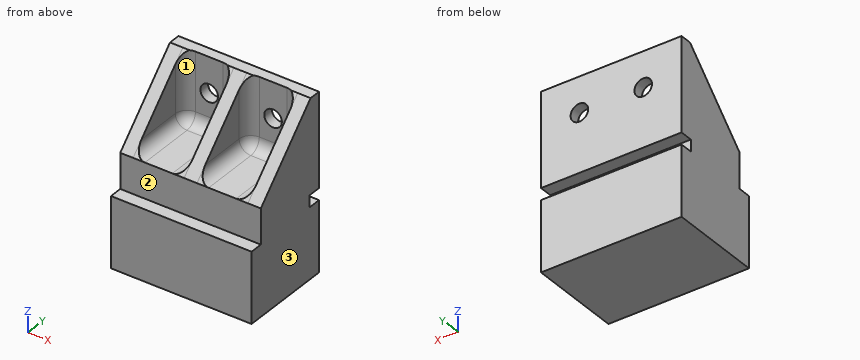
from build123d import *

# Parameters (mm, degrees)
F1_DEPTH     = 38.1
F2_W         = 13.81125
F2_H         = 19.05
F3_DEPTH     = 19.05
F4_T1_DEPTH  = 7.46125
F4_T3_DEPTH  = 7.46125
F4_S7_W      = 3.175
F4_S7_H      = 3.175
F4_T8_DEPTH  = 3.175
F4_S13_W     = 3.175
F4_S13_H     = 3.175
F4_T14_DEPTH = 3.175
F4_S19_W     = 3.175
F4_S19_H     = 3.175
F4_T20_DEPTH = 3.175
F4_S25_W     = 3.175
F4_S25_H     = 3.175
F4_T26_DEPTH = 3.175
F4_T32_DEPTH = 15.875
F4_T37_DEPTH = 15.875
F4_T42_DEPTH = 15.875
F4_T47_DEPTH = 15.875
F4_T52_DEPTH = 15.875
F4_T57_DEPTH = 15.875
F4_T62_DEPTH = 15.875
F4_T67_DEPTH = 15.875
F6_DEPTH     = 2.8585


# Not quite as in the source:
# - a fillet or chamfer that OpenCascade refuses, or shapes differently, is made with other operations: its cross-section is extruded or revolved along the edge and cut away or added


with BuildPart() as f1:
    # F0 (on Right) → F1 (new body)
    with BuildSketch(Plane.YZ):
        Polygon((0, 19.05), (0, 0), (25.4, 0), (25.4, 19.05), (21.9075, 19.05), (21.9075, 22.225), (25.4, 22.225), (25.4, 47.625), (22.225, 47.625), (22.225, 28.575), (3.4925, 28.575), (3.4925, 19.05), align=None)
        Polygon((22.225, 47.625), (3.4925, 28.575), (22.225, 28.575), align=None)
    extrude(amount=F1_DEPTH)

    # F2 (on face) → F3 (cut)
    with BuildSketch(Plane.XZ.offset(-3.4925)):
        with Locations((27.701875, 38.1)):
            Rectangle(F2_W, F2_H)
        with Locations((10.398125, 38.1)):
            Rectangle(F2_W, F2_H)
    extrude(amount=-F3_DEPTH, mode=Mode.SUBTRACT)

    # F4: fillet of radius 3.175 on 10 edges, made by hand

    # F4_s2 → F4_t1 (join)
    with BuildSketch(Plane.YZ.offset(6.6675)):
        with BuildLine():
            ThreePointArc((19.3675, 28.575), (21.6125640303, 29.5049359697), (22.5425, 31.75))
            Line((22.5425, 31.75), (22.5425, 28.575))
            Line((22.5425, 28.575), (19.3675, 28.575))
        make_face()
    extrude(amount=F4_T1_DEPTH)

    # F4_s4 → F4_t3 (join)
    with BuildSketch(Plane.YZ.offset(23.97125)):
        with BuildLine():
            ThreePointArc((19.3675, 28.575), (21.6125640303, 29.5049359697), (22.5425, 31.75))
            Line((22.5425, 31.75), (22.5425, 28.575))
            Line((22.5425, 28.575), (19.3675, 28.575))
        make_face()
    extrude(amount=F4_T3_DEPTH)


with BuildPart() as f4_tool6:
    # F4_s7 → F4_t8 (new body)
    with BuildSketch(Plane.YZ.offset(6.6675)):
        with Locations((20.955, 30.1625)):
            Rectangle(F4_S7_W, F4_S7_H)
    extrude(amount=-F4_T8_DEPTH)

    # F4_s9 → F4_t10 (revolve, cut)
    with BuildSketch(Plane(origin=(6.6675, 19.3675, 31.75), x_dir=(0, -0.7071067812, 0.7071067812), z_dir=(0, -0.7071067812, -0.7071067812))):
        with BuildLine():
            ThreePointArc((0, -3.175), (3.175, 0), (0, 3.175))
            Line((0, 3.175), (0, -3.175))
        make_face()
    revolve(axis=Axis((6.6675, 19.3675, 31.75), (-1, 0, 0)), mode=Mode.SUBTRACT)


with BuildPart() as f1_1:
    add(f1.part)

    # F4_t5: union F4_tool6
    add(f4_tool6.part)


with BuildPart() as f4_tool12:
    # F4_s13 → F4_t14 (new body)
    with BuildSketch(Plane.XZ.offset(-19.3675)):
        with Locations((15.71625, 30.1625)):
            Rectangle(F4_S13_W, F4_S13_H)
    extrude(amount=-F4_T14_DEPTH)

    # F4_s15 → F4_t16 (revolve, cut)
    with BuildSketch(Plane(origin=(14.12875, 19.3675, 31.75), x_dir=(-0.7071067812, 0, 0.7071067812), z_dir=(-0.7071067812, 0, -0.7071067812))):
        with BuildLine():
            ThreePointArc((0, -3.175), (3.175, 0), (0, 3.175))
            Line((0, 3.175), (0, -3.175))
        make_face()
    revolve(axis=Axis((14.12875, 19.3675, 31.75), (0, 1, 0)), mode=Mode.SUBTRACT)


with BuildPart() as f1_2:
    add(f1_1.part)

    # F4_t11: union F4_tool12
    add(f4_tool12.part)


with BuildPart() as f4_tool18:
    # F4_s19 → F4_t20 (new body)
    with BuildSketch(Plane.XY.offset(31.75)):
        with Locations((22.38375, 20.955)):
            Rectangle(F4_S19_W, F4_S19_H)
    extrude(amount=-F4_T20_DEPTH)

    # F4_s21 → F4_t22 (revolve, cut)
    with BuildSketch(Plane(origin=(23.97125, 19.3675, 31.75), x_dir=(0.7071067812, -0.7071067812, 0), z_dir=(0.7071067812, 0.7071067812, 0))):
        with BuildLine():
            ThreePointArc((0, -3.175), (3.175, 0), (0, 3.175))
            Line((0, 3.175), (0, -3.175))
        make_face()
    revolve(axis=Axis((23.97125, 19.3675, 31.75), (0, 0, -1)), mode=Mode.SUBTRACT)


with BuildPart() as f1_3:
    add(f1_2.part)

    # F4_t17: union F4_tool18
    add(f4_tool18.part)


with BuildPart() as f4_tool24:
    # F4_s25 → F4_t26 (new body)
    with BuildSketch(Plane.XY.offset(31.75)):
        with Locations((33.02, 20.955)):
            Rectangle(F4_S25_W, F4_S25_H)
    extrude(amount=-F4_T26_DEPTH)

    # F4_s27 → F4_t28 (revolve, cut)
    with BuildSketch(Plane(origin=(31.4325, 19.3675, 31.75), x_dir=(-0.7071067812, -0.7071067812, 0), z_dir=(0.7071067812, -0.7071067812, 0))):
        with BuildLine():
            ThreePointArc((0, -3.175), (3.175, 0), (0, 3.175))
            Line((0, 3.175), (0, -3.175))
        make_face()
    revolve(axis=Axis((31.4325, 19.3675, 31.75), (0, 0, -1)), mode=Mode.SUBTRACT)


with BuildPart() as f1_4:
    add(f1_3.part)

    # F4_t23: union F4_tool24
    add(f4_tool24.part)


with BuildPart() as f4_tool30:
    # F4_s31 → F4_t32 (new body)
    with BuildSketch(Plane.XY.offset(47.625)):
        with BuildLine():
            ThreePointArc((20.79625, 19.3675), (21.7261859697, 21.6125640303), (23.97125, 22.5425))
            Line((23.97125, 22.5425), (20.79625, 22.5425))
            Line((20.79625, 22.5425), (20.79625, 19.3675))
        make_face()
    extrude(amount=-F4_T32_DEPTH)

    split(bisect_by=Plane(origin=(0, -12.5098856094, 12.3013875159), x_dir=(1, 0, 0), z_dir=(0, 0.7130236798, -0.7011399518)), keep=Keep.TOP)


with BuildPart() as f1_5:
    add(f1_4.part)

    # F4_t29: union F4_tool30
    add(f4_tool30.part)


with BuildPart() as f4_tool35:
    # F4_s36 → F4_t37 (new body)
    with BuildSketch(Plane.XZ.offset(-3.4925)):
        with BuildLine():
            ThreePointArc((23.97125, 28.575), (21.7261859697, 29.5049359697), (20.79625, 31.75))
            Line((20.79625, 31.75), (20.79625, 28.575))
            Line((20.79625, 28.575), (23.97125, 28.575))
        make_face()
    extrude(amount=-F4_T37_DEPTH)

    split(bisect_by=Plane(origin=(0, -12.5098856094, 12.3013875159), x_dir=(1, 0, 0), z_dir=(0, 0.7130236798, -0.7011399518)), keep=Keep.TOP)


with BuildPart() as f1_6:
    add(f1_5.part)

    # F4_t34: union F4_tool35
    add(f4_tool35.part)


with BuildPart() as f4_tool40:
    # F4_s41 → F4_t42 (new body)
    with BuildSketch(Plane.XY.offset(47.625)):
        with BuildLine():
            ThreePointArc((3.4925, 19.3675), (4.4224359697, 21.6125640303), (6.6675, 22.5425))
            Line((6.6675, 22.5425), (3.4925, 22.5425))
            Line((3.4925, 22.5425), (3.4925, 19.3675))
        make_face()
    extrude(amount=-F4_T42_DEPTH)

    split(bisect_by=Plane(origin=(0, -12.5098856094, 12.3013875159), x_dir=(1, 0, 0), z_dir=(0, 0.7130236798, -0.7011399518)), keep=Keep.TOP)


with BuildPart() as f1_7:
    add(f1_6.part)

    # F4_t39: union F4_tool40
    add(f4_tool40.part)


with BuildPart() as f4_tool45:
    # F4_s46 → F4_t47 (new body)
    with BuildSketch(Plane.XZ.offset(-3.4925)):
        with BuildLine():
            ThreePointArc((6.6675, 28.575), (4.4224359697, 29.5049359697), (3.4925, 31.75))
            Line((3.4925, 31.75), (3.4925, 28.575))
            Line((3.4925, 28.575), (6.6675, 28.575))
        make_face()
    extrude(amount=-F4_T47_DEPTH)

    split(bisect_by=Plane(origin=(0, -12.5098856094, 12.3013875159), x_dir=(1, 0, 0), z_dir=(0, 0.7130236798, -0.7011399518)), keep=Keep.TOP)


with BuildPart() as f1_8:
    add(f1_7.part)

    # F4_t44: union F4_tool45
    add(f4_tool45.part)


with BuildPart() as f4_tool50:
    # F4_s51 → F4_t52 (new body)
    with BuildSketch(Plane.XZ.offset(-3.4925)):
        with BuildLine():
            ThreePointArc((31.4325, 28.575), (33.6775640303, 29.5049359697), (34.6075, 31.75))
            Line((34.6075, 31.75), (34.6075, 28.575))
            Line((34.6075, 28.575), (31.4325, 28.575))
        make_face()
    extrude(amount=-F4_T52_DEPTH)

    split(bisect_by=Plane(origin=(0, -12.5098856094, 12.3013875159), x_dir=(1, 0, 0), z_dir=(0, 0.7130236798, -0.7011399518)), keep=Keep.TOP)


with BuildPart() as f1_9:
    add(f1_8.part)

    # F4_t49: union F4_tool50
    add(f4_tool50.part)


with BuildPart() as f4_tool55:
    # F4_s56 → F4_t57 (new body)
    with BuildSketch(Plane.XY.offset(31.75)):
        with BuildLine():
            ThreePointArc((31.4325, 22.5425), (33.6775640303, 21.6125640303), (34.6075, 19.3675))
            Line((34.6075, 19.3675), (34.6075, 22.5425))
            Line((34.6075, 22.5425), (31.4325, 22.5425))
        make_face()
    extrude(amount=F4_T57_DEPTH)

    split(bisect_by=Plane(origin=(0, -12.5098856094, 12.3013875159), x_dir=(1, 0, 0), z_dir=(0, 0.7130236798, -0.7011399518)), keep=Keep.TOP)


with BuildPart() as f1_10:
    add(f1_9.part)

    # F4_t54: union F4_tool55
    add(f4_tool55.part)


with BuildPart() as f4_tool60:
    # F4_s61 → F4_t62 (new body)
    with BuildSketch(Plane.XZ.offset(-3.4925)):
        with BuildLine():
            ThreePointArc((14.12875, 28.575), (16.3738140303, 29.5049359697), (17.30375, 31.75))
            Line((17.30375, 31.75), (17.30375, 28.575))
            Line((17.30375, 28.575), (14.12875, 28.575))
        make_face()
    extrude(amount=-F4_T62_DEPTH)

    split(bisect_by=Plane(origin=(0, -12.5098856094, 12.3013875159), x_dir=(1, 0, 0), z_dir=(0, 0.7130236798, -0.7011399518)), keep=Keep.TOP)


with BuildPart() as f1_11:
    add(f1_10.part)

    # F4_t59: union F4_tool60
    add(f4_tool60.part)


with BuildPart() as f4_tool65:
    # F4_s66 → F4_t67 (new body)
    with BuildSketch(Plane.XY.offset(31.75)):
        with BuildLine():
            ThreePointArc((14.12875, 22.5425), (16.3738140303, 21.6125640303), (17.30375, 19.3675))
            Line((17.30375, 19.3675), (17.30375, 22.5425))
            Line((17.30375, 22.5425), (14.12875, 22.5425))
        make_face()
    extrude(amount=F4_T67_DEPTH)

    split(bisect_by=Plane(origin=(0, -12.5098856094, 12.3013875159), x_dir=(1, 0, 0), z_dir=(0, 0.7130236798, -0.7011399518)), keep=Keep.TOP)


with BuildPart() as f1_12:
    add(f1_11.part)

    # F4_t64: union F4_tool65
    add(f4_tool65.part)

    # F5 (on face) → F6 (cut, through all)
    with BuildSketch(Plane.XZ.offset(-22.5425)):
        with BuildLine():
            ThreePointArc((10.398125, 35.71875), (12.0819230227, 36.4162019773), (12.779375, 38.1))
            ThreePointArc((12.779375, 38.1), (8.7143269773, 39.7837980227), (10.398125, 35.71875))
        make_face()
        with BuildLine():
            ThreePointArc((27.701875, 35.71875), (29.3856730227, 36.4162019773), (30.083125, 38.1))
            ThreePointArc((30.083125, 38.1), (26.0180769773, 39.7837980227), (27.701875, 35.71875))
        make_face()
    extrude(amount=-F6_DEPTH, mode=Mode.SUBTRACT)


solid = f1_12.part
Here's how the part is built. I have some questions about the finished solid (model axes, mm). Face numbers are marked on the shaded views. A direction names the side the tool comes from. Round coordinates to 2 decimals unless told otherwise and drop trailing zeros. Order: outer loops, then holes, each group sorted by start corner. A loop starts at its lowest first (then second) coordinate and runs counter-clockwise, first axis right, second up. Notation, with made-up numbers: M 5.5,47 L 49.5,47 A24 cw 49.5,65 Z; hole C 76,67.25 d5. An arc over 180 degrees is marked long. One line per question, with ' | ' between items.
1) Imagine slicing it at A-A, the plane y = 23.25. Count the separate pieces of the cut face and the enclosed holes in it, plus the area to 3 significant figures.
Checked values:
separate pieces: 2 | enclosed holes: 2 | area: 1,660 mm²
2) I'm going to push flat-ended pins straight in: pin 1 Ø8 at (x, z) = (9, 38.5) entering from -Y; pin 2 Ø8 at (x, y) = (10, 10.5) entering from +Z; pin 3 Ø8 at (x, y) = (8, 10.5) entering from +Z. Where does each tip first touch, or does it pass through?
Checked values:
pin 1: stops at y = 22.07 | pin 2: stops at z = 28.65 | pin 3: stops at z = 30.03
3) Imagine slicing it at D-D, the plane z = 30.5. Write out the boundary of the cut face in (x, y).
Checked values:
outline: M 0,5.39 L 3.75,5.39 L 3.75,19.37 A2.92 cw 6.67,22.29 L 14.13,22.29 A2.92 cw 17.05,19.37 L 17.05,5.39 L 21.05,5.39 L 21.05,19.37 A2.92 cw 23.97,22.29 L 31.43,22.29 A2.92 cw 34.35,19.37 L 34.35,5.39 L 38.1,5.39 L 38.1,25.4 L 0,25.4 Z
4) I need wall thicknesses on line 1 (X direction, y = 18, z = 35.5); line 2 (X direction, y = 23.3, z = 38.1); line 3 (Z direction, x = 33.5, y = 2). Which ranges of each line are inside material? Lowest first, please.
Checked values:
line 1: x = 0 to 3.49, 17.3 to 20.8, 34.61 to 38.1 | line 2: x = 0 to 8.02, 12.78 to 25.32, 30.08 to 38.1 | line 3: z = 0 to 19.05
5) On a 3-axis mill with a long thin cutter (end or side, diameter ignored), from which of +Z, -Z, +X, -X, +Y, -Y can I reach the whole of each face in a straight line? I mean the marked faces 1, 2 and 3. Say none if no direction works.
Checked values:
face 1: +Z, -Y | face 2: +Z, +X, -X, -Y | face 3: +Z, -Z, +X, +Y, -Y
